Verification items for the finished model (mm, model axes). A direction names the side the tool comes from. Coordinates: 2 decimals unless noted, no trailing zeros. Order: outer loops, then holes, each group sorted by start corner. A loop starts at its lowest first (then second) coordinate and runs counter-clockwise, first axis right, second up. Notation, with made-up numbers: (-40, 80.25) -> (13, 80.25) arc R28 cw to (13, 109.25) -> close; hole circle Ø8 at (7.5, -3). An arc over 180 degrees is marked (long way). Write item = value, one per line. Start each with the question number.
1. Set-up check for faces 4 (the cylindrical face through (-86.198, -5.455, 20.493)), 5 (the flat face through (284.472, -23, 10)): record each of +Z, -Z, +X, -X, +Y, -Y from which the full face is reachable in a straight line by a thin tool's end or side.
2. Cross-section at D-D on y = -66. Record the cut outline in (x, z), plus the area to 3 significant figures.
3. Cross-section at C-C on x = 217. Record the cut outline in (y, z).
4. Go/stop test with a flat-tipped pin: P1, Ø4, axis at x = 78.5, y = -85.5, coming from the +Z side. Record where the tip stops, or that it passes through.
5. Thickness scan on line 1 along X through (y, z) = (-16, 14); line 2 along Z through (x, y) = (-176, -56); line 3 along X through (y, z) = (55.5, 12). Record the ranges inside material, lowest first. Write a range as from..to.
6. Cross-section at A-A on y = -40. Record the cut outline in (x, z), plus the area to 3 significant figures.
7. Release check for a two-part mould opening along Y. For faces 1 (the flat face through (-116, -15, 45)), 2 (the flat face through (-116, -21, 20)), 3 (the cylindrical face through (-140.923, -34.163, 20.493)) record: +Y half, -Y half, draft (parallel to the pull), parting line (faces both ways), or undercut.
8. Cross-section at B-B on z = 13.5. Give the number of separate pieces and of enclosed holes in the cut face, plus the area to 3 significant figures.
from build123d import *

# Parameters (mm, degrees)
F0_R     = 15
F0_R_2   = 32
F0_R_3   = 30.75
F0_R_4   = 5
F1_DEPTH = 20
F2_DEPTH = 21
F3_DEPTH = 45


with BuildPart() as f1:
    # F0 (on Top) → F1 (new body)
    with BuildSketch(Plane.XY):
        Polygon((284.4715710252, 88.1958252929), (-215.5284289748, 88.1958252929), (-215.5284289748, -14.6917872616), (-215.5284289748, -112.5681422158), (-215.5284289748, -131.8041747071), (284.4715710252, -131.8041747071), (284.4715710252, -112.5681422158), align=None)
        with Locations((77.0776277755, -29.4956769794)):
            Circle(F0_R, mode=Mode.SUBTRACT)
        with Locations((-115.5284289748, -14.6917872616)):
            Circle(F0_R_2, mode=Mode.SUBTRACT)
        with Locations((62.4715710252, 4.5043230206)):
            Circle(F0_R, mode=Mode.SUBTRACT)
        with Locations((111.0776277755, -11.4509115215)):
            Circle(F0_R, mode=Mode.SUBTRACT)
        with Locations((145.0776277755, -0.0014326224)):
            Circle(F0_R, mode=Mode.SUBTRACT)
        with Locations((96.4715710252, 22.5490884785)):
            Circle(F0_R, mode=Mode.SUBTRACT)
        with Locations((179.0776277755, 8.3279051832)):
            Circle(F0_R, mode=Mode.SUBTRACT)
        with Locations((130.4715710252, 33.9985673776)):
            Circle(F0_R, mode=Mode.SUBTRACT)
        with Locations((164.4715710252, 42.3279051832)):
            Circle(F0_R, mode=Mode.SUBTRACT)
        with Locations((-115.5284289748, -14.6917872616)):
            Circle(F0_R_2)
        with Locations((-115.5284289748, -14.6917872616)):
            Circle(F0_R_3, mode=Mode.SUBTRACT)
        with Locations((-115.5284289748, -14.6917872616)):
            Circle(F0_R_3)
        with Locations((-115.5284289748, -14.6917872616)):
            Circle(F0_R_4, mode=Mode.SUBTRACT)
        with Locations((-115.5284289748, -14.6917872616)):
            Circle(F0_R_4)
    extrude(amount=F1_DEPTH)

    # F0 (on Top) → F2 (join)
    with BuildSketch(Plane.XY):
        with Locations((-115.5284289748, -14.6917872616)):
            Circle(F0_R_2)
        with Locations((-115.5284289748, -14.6917872616)):
            Circle(F0_R_3, mode=Mode.SUBTRACT)
    extrude(amount=F2_DEPTH)

    # F0 (on Top) → F3 (join)
    with BuildSketch(Plane.XY):
        with Locations((-115.5284289748, -14.6917872616)):
            Circle(F0_R_4)
    extrude(amount=F3_DEPTH)


solid = f1.part
Worked out:
q1.face_4 = +Z
q1.face_5 = +Z, -Z, +X, +Y, -Y
q2.outline = (-215.53, 0) -> (284.47, 0) -> (284.47, 20) -> (-215.53, 20) -> close
q2.area = 10,000 mm²
q3.outline = (-131.8, 0) -> (88.2, 0) -> (88.2, 20) -> (-131.8, 20) -> close
q4.P1 = 20
q5.line_1 = -215.53..70.53, 83.62..96.78, 125.37..284.47
q5.line_2 = 0..20
q5.line_3 = -215.53..157.3, 171.65..284.47
q6.outline = (-215.53, 0) -> (66.37, 0) -> (66.37, 20) -> (-95.95, 20) -> (-95.95, 21) -> (-98.06, 21) -> (-98.06, 20) -> (-132.99, 20) -> (-132.99, 21) -> (-135.11, 21) -> (-135.11, 20) -> (-215.53, 20) -> close; (87.79, 0) -> (284.47, 0) -> (284.47, 20) -> (87.79, 20) -> close
q6.area = 9,580 mm²
q7.face_1 = draft
q7.face_2 = undercut
q7.face_3 = parting line
q8.separate_pieces = 1
q8.enclosed_holes = 8
q8.area = 104,000 mm²
